CAD build for the part. Positions are in the model's coordinates, mm. Round coordinates to 2 decimals unless told otherwise and drop trailing zeros. Loops run counter-clockwise (first coordinate to the right, second up) from the corner with the lowest first, then second, coordinate; pieces in that order, holes last. Notation, with made-up numbers: M -5.5,-18 L 43.5,-18 A20 ccw 43.5,15 Z; hole C 43,33 d2. An arc over 180 degrees is marked long. Use a Markdown table: item, result. Add a question column.
(1) Band-saw the part on A-A, the plane y = -37. Write the cut outline in (x, z).
(2) Band-saw the part on B-B, the plane y = 15. Write the cut outline in (x, z).
(3) Band-saw the part on D-D, the plane y = 59. Write the cut outline in (x, z).
(4) Wall check: L1, parallel to Y at x = -75.5, z = 0.95; L2, parallel to Y at x = 32.5, z = 0.65; L3, parallel to Y at x = -61, z = 0.3. Give the ranges that are in metal, low to high.
(5) Band-saw the part on C-C, the plane x = 27.5. Write the cut outline in (y, z).
(6) Two-plate mould, pull along X, no slides. Class faces 1 (the face through (-2, 1, 1)), 2 (the face through (31.045, 39.939, 0.507)), 3 (the face through (-45.28, 20.87, 0.51)): released by +X, released by -X, zero draft, split by the parting line, or undercut.
from build123d import *

# Parameters (mm, degrees)
SKETCH_1_W          = 216
SKETCH_1_H          = 200
EXTRUDE_1_DEPTH     = 1
CUT_EXTRUDE_2_DEPTH = 148.190352945
CUT_EXTRUDE_3_DEPTH = 148.190352945
SKETCH_4_W          = 26.549290854
SKETCH_4_H          = 6.938085034
CUT_EXTRUDE_4_DEPTH = 148.190352945


with BuildPart() as part:
    # 草图1 → 凸台-拉伸1 (new body)
    with BuildSketch(Plane.XY):
        Rectangle(SKETCH_1_W, SKETCH_1_H)
    extrude(amount=EXTRUDE_1_DEPTH)

    # 草图2 → 切除-拉伸2 (cut, through all)
    with BuildSketch(Plane.XY.offset(1)):
        Polygon((-29.908359309, 82.116750483), (0, 52.560653053), (29.908359309, 82.116750483), (16.210763117, 82.116750483), (0, 65.905987366), (-16.210763117, 82.116750483), align=None)
        Polygon((0, 26.550736561), (-45.925349273, 72.476085834), (-63.582203523, 72.476085834), (0, 8.893882312), (62.972238909, 71.866121221), (45.31538466, 71.866121221), align=None)
    cut_extrude_2 = extrude(amount=-CUT_EXTRUDE_2_DEPTH, mode=Mode.SUBTRACT)

    # 镜向2: 切除-拉伸2 across plane
    add(cut_extrude_2.mirror(Plane.ZX), mode=Mode.SUBTRACT)

    # 草图3 → 切除-拉伸3 (cut, through all)
    with BuildSketch(Plane.XY.offset(1)):
        Polygon((-46.068138611, 0), (-65.582203523, 19.514064912), (-65.582203523, 41.170919161), (-24.411284361, 0), (-65.582203523, -41.170919161), (-65.582203523, -19.514064912), align=None)
    cut_extrude_3 = extrude(amount=-CUT_EXTRUDE_3_DEPTH, mode=Mode.SUBTRACT)

    # 镜向3: 切除-拉伸3 across plane
    add(cut_extrude_3.mirror(Plane(origin=(0, 0, 0), x_dir=(0, 0, 1), z_dir=(1, 0, 0))), mode=Mode.SUBTRACT)

    # 草图4 → 切除-拉伸4 (cut, through all)
    with BuildSketch(Plane.XY.offset(1)):
        with Locations((-83.979598966, 16.045022395)):
            Rectangle(SKETCH_4_W, SKETCH_4_H)
    cut_extrude_4 = extrude(amount=-CUT_EXTRUDE_4_DEPTH, mode=Mode.SUBTRACT)

    # 镜向4: 切除-拉伸4 across plane
    add(cut_extrude_4.mirror(Plane(origin=(0, 0, 0), x_dir=(0, 0, 1), z_dir=(1, 0, 0))), mode=Mode.SUBTRACT)


solid = part.part
Return value:
| question | item | result |
|---|---|---|
| 1 | outline | M -108,0 L -65.58,0 L -65.58,1 L -108,1 Z; M -61.41,0 L -28.11,0 L -28.11,1 L -61.41,1 Z; M -10.45,0 L 10.45,0 L 10.45,1 L -10.45,1 Z; M 28.11,0 L 61.41,0 L 61.41,1 L 28.11,1 Z; M 65.58,0 L 108,0 L 108,1 L 65.58,1 Z |
| 2 | outline | M -108,0 L -97.25,0 L -97.25,1 L -108,1 Z; M -70.7,0 L -61.07,0 L -61.07,1 L -70.7,1 Z; M -39.41,0 L -6.11,0 L -6.11,1 L -39.41,1 Z; M 6.11,0 L 39.41,0 L 39.41,1 L 6.11,1 Z; M 61.07,0 L 70.7,0 L 70.7,1 L 61.07,1 Z; M 97.25,0 L 108,0 L 108,1 L 97.25,1 Z |
| 3 | outline | M -108,0 L -50.11,0 L -50.11,1 L -108,1 Z; M -32.45,0 L -6.52,0 L -6.52,1 L -32.45,1 Z; M 6.52,0 L 32.45,0 L 32.45,1 L 6.52,1 Z; M 50.11,0 L 108,0 L 108,1 L 50.11,1 Z |
| 4 | L1 | -100 to 12.58, 19.51 to 100 |
| 4 | L2 | -100 to -59.05, -41.39 to -8.09, 8.09 to 41.39, 59.05 to 100 |
| 4 | L3 | -100 to -72.48, -69.89 to -36.59, -14.93 to 14.93, 36.59 to 69.89, 72.48 to 100 |
| 5 | outline | M -100,0 L -82.12,0 L -82.12,1 L -100,1 Z; M -79.74,0 L -54.05,0 L -54.05,1 L -79.74,1 Z; M -36.39,0 L -3.09,0 L -3.09,1 L -36.39,1 Z; M 3.09,0 L 36.39,0 L 36.39,1 L 3.09,1 Z; M 54.05,0 L 79.74,0 L 79.74,1 L 54.05,1 Z; M 82.12,0 L 100,0 L 100,1 L 82.12,1 Z |
| 6 | face 1 | zero draft |
| 6 | face 2 | undercut |
| 6 | face 3 | undercut |
